The listing builds one solid part. Answer for the finished solid, in the listing's coordinates (mm). Face numbers are marked on the shaded views. A direction names the side the tool comes from. Coordinates: 2 decimals unless noted, no trailing zeros. Order: outer loops, then holes, each group sorted by start corner. A loop starts at its lowest first (then second) coordinate and runs counter-clockwise, first axis right, second up.
Autodesk Inventor part; units mm, degrees
ref_plane "Work Plane1" through (5.2, 0, 0) normal (1, 0, 0) x (0, 1, 0)
ref_plane "Work Plane2" through (0, 0, 5.2) normal (0, 0, 1) x (1, 0, 0)
ref_plane "XZ Plane" through (0, 0, 0) normal (0, 1, 0) x (-1, 0, 0)
sketch "Sketch2" plane through (0, 0, 0) normal (0, 0, 1) x (1, 0, 0)
  line L0 (0, 4.1785) -> (1.6, 4.1785)
  line L1 (1.6, 4.1785) -> (1.6, 5.6785)
  line L2 (1.6, 5.6785) -> (2.5, 5.6785)
  line L3 (2.5, 5.6785) -> (2.5, 4.1785)
  line L4 (2.5, 4.1785) -> (3.2, 4.1785)
  arc A0 (5.2, 2.1785) -> (3.2, 4.1785) centre (3.2, 2.1785) ccw
  line L5 (5.2, 2.1785) -> (5.2, -2.1785)
  arc A1 (3.157, -4.2215) -> (5.2, -2.1785) centre (3.157, -2.1785) ccw
  line L6 (3.157, -4.2215) -> (3.157, -5.4215)
  line L7 (3.157, -5.4215) -> (2.5, -5.4215)
  line L8 (2.5, -5.4215) -> (2.5, 2.5785)
  line L9 (2.5, 2.5785) -> (0, 2.5785)
  line L10 (0, 2.5785) -> (0, 4.1785)
  point P0 (0, 0)
  point P1 (5.2, 0)
  dimension "d0" = 5
  dimension "d1" = 3.2
  dimension "d2" = 1.5
  dimension "d3" = 2
  dimension "d4" = 10.4
  dimension "d6" = 6.314
  dimension "d7" = 1.2
  dimension "d8" = 8
  dimension "d23" = 9.6
revolve "Revolution1" add sketch "Sketch2" angle 360 about axis through (0, 2.5785, 0) along (0, 1, 0)
sketch "Sketch3" plane through (0, 4.1785, 0) normal (0, 1, 0) x (1, 0, 0)
  circle A0 centre (0, 0) radius 1.6
  line L0 (-0.4, 1.5492) -> (-0.4, 0.2309)
  line L1 (-0.4, 0.2309) -> (-1.5416, -0.4282)
  line L2 (-1.1416, -1.121) -> (0, -0.4619)
  line L3 (0, -0.4619) -> (1.1416, -1.121)
  line L4 (1.5416, -0.4282) -> (0.4, 0.2309)
  line L5 (0.4, 0.2309) -> (0.4, 1.5492)
  dimension "d10" = 120
  dimension "d11" = 0.8
extrude "Extrusion1" cut sketch "Sketch3" against normal through all contours A0 L4 L5 | L0 L1 A0 | A0 L2 L3
fillet "Fillet1" radius 0.1 2 edges at (-2.5, 5.6785, 0) (-3.157, -5.4215, 0)
ref_plane "Work Plane1" through (5.2, 0, 0) normal (1, 0, 0) x (0, 1, 0)
ref_plane "Work Plane2" through (0, 0, 5.2) normal (0, 0, 1) x (1, 0, 0)
sketch "Sketch5" plane through (0, 0, 5.2) normal (0, 0, 1) x (1, 0, 0)
  line L0 (-5.2, 2.1785) -> (5.2, 2.1785) construction
  line L1 (-5.2, -2.1785) -> (5.2, -2.1785) construction
  line L2 (-5.8921, 2.1785) -> (5.8921, 2.1785) construction
  line L3 (5.8921, 2.1785) -> (5.8921, -2.1785) construction
  line L4 (5.8921, -2.1785) -> (-5.8921, -2.1785) construction
  line L5 (-5.8921, -2.1785) -> (-5.8921, 2.1785) construction
  point P0 (0, 0)
  point P1 (0, 2.1785)
decal "Decal2"
properties part number "X02598_LEGOmini_Head_Y_Original_NoPara" material "ABS Plastic"
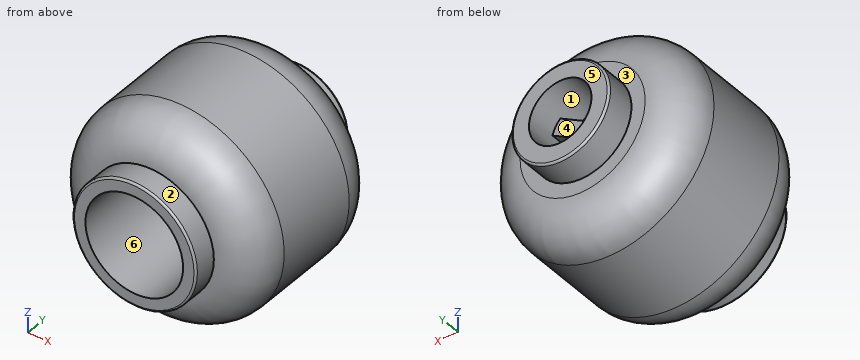
(1) Find section A-A (z = 0). Give the number of separate pieces and of enclosed holes in the cut face, and give its area (3 significant figures).
(2) Find section C-C (y = -4.5). Write down the section's boundary in (x, z), and give its area (3 significant figures).
(3) For the marked faces 4, 5 and 6, determine the directions among +Z, -Z, +X, -X, +Y, -Y from which every point of the face is accessible in a straight line to the end or side of a thin tool.
(4) Consider line 1 (X direction, y = 4.9, z = 0); line 2 (X direction, y = 4, z = 0). Determine where each line is inside the solid, lowest interval first.
(5) Find section D-D (y = -3.25). Write down the section's boundary in (x, z).
(6) The mould has two halves that part along X. Classify the marked faces 1, 2 and 3: released by +X, released by -X, zero draft, split by the parting line, or undercut.
(7) Find section B-B (y = 2.75). Write down the section's boundary in (x, z).
(8) Each of these flat-tipped pins is pushed along its axis until it touches: pin 1 Ø1.1 at (y, z) = (3.5, -1) entering from +X; pin 2 Ø1.9 at (x, z) = (0, 0) entering from +Y; pin 3 Ø0.7 at (y, z) = (3.5, -1) entering from -X. Where does it stop, or does it pass through?
Findings below:
1. separate pieces: 3
1. enclosed holes: 0
1. area: 51.6 mm2
2. outline: circle Ø6.31 at (0, 0); hole circle Ø5 at (0, 0)
2. area: 11.7 mm2
3. face 4: +Y
3. face 5: +Z, -Z, +X, -X, +Y
3. face 6: -Y
4. line 1: x = -2.5 to -1.6, 1.6 to 2.5
4. line 2: x = -4.03 to -1.6, -0.8 to 0.8, 1.6 to 4.03
5. outline: circle Ø9.79 at (0, 0); hole circle Ø5 at (0, 0)
6. face 1: undercut
6. face 2: split by the parting line
6. face 3: zero draft
7. outline: circle Ø10.23 at (0, 0); hole (-1.54, 0.43) arc R1.6 ccw to (-0.4, -1.55) - (-0.4, -0.23) - close; hole (-1.14, 1.12) - (0, 0.46) - (1.14, 1.12) arc R1.6 ccw to start; hole (0.4, -1.55) arc R1.6 ccw to (1.54, 0.43) - (0.4, -0.23) - close
8. pin 1: stops at x = 4.97
8. pin 2: stops at y = 4.18
8. pin 3: stops at x = -4.86
